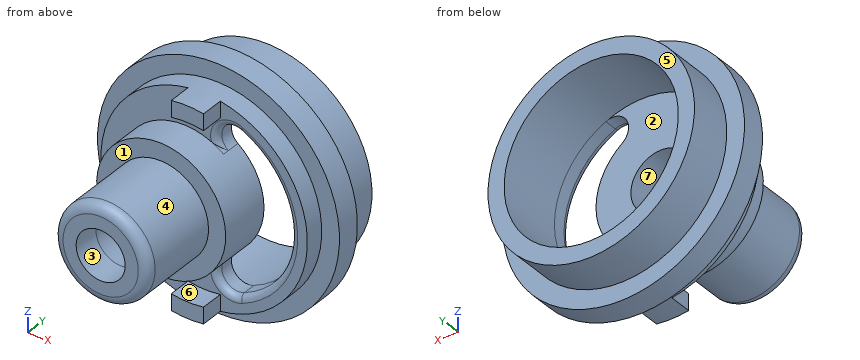
from build123d import *

# Parameters (mm, degrees)
SKETCH1_R              = 8.128
TOP_BODY_DEPTH         = 6.858
SKETCH2_R              = 5.08
ECCENTRIC_SLEEVE_DEPTH = 2.54
SKETCH3_R              = 3.724670389
ECCENTRIC_SHAFT_DEPTH  = 15.8242
SKETCH4_R              = 9.525
FLANGE_DEPTH           = 1.905
SKETCH5_R              = 6.858
TOP_HOLE_DEPTH         = 18.073240643
GROOVE_DEPTH           = 18.073240643
PINS_DEPTH             = 1.778
FILLET1_R              = 0.508
FILLET2_R              = 0.762


with BuildPart() as part:
    # Sketch1 → Top Body (new body)
    with BuildSketch(Plane(origin=(0, 0, 0), x_dir=(1, 0, 0), z_dir=(0, 1, 0))):
        with Locations(Location((0, 0, 0), (0, 0, 270))):
            Circle(SKETCH1_R)
    extrude(amount=TOP_BODY_DEPTH)

    # Sketch2 → Eccentric Sleeve (add)
    with BuildSketch(Plane.XZ):
        with Locations(Location((-1.4986, 0, 0), (0, 0, 90))):
            Circle(SKETCH2_R)
    extrude(amount=ECCENTRIC_SLEEVE_DEPTH)

    # Sketch3 → Eccentric Shaft (add)
    with BuildSketch(Plane(origin=(0, 6.858, 0), x_dir=(-1, 0, 0), z_dir=(0, 1, 0))):
        with Locations(Location((1.4986, 0, 0), (0, 0, 90))):
            Circle(SKETCH3_R)
    extrude(amount=-ECCENTRIC_SHAFT_DEPTH)

    # Sketch4 → Flange (add)
    with BuildSketch(Plane.XZ.offset(-1.524)):
        with Locations(Location((0, 0, 0), (0, 0, 270))):
            Circle(SKETCH4_R)
    extrude(amount=-FLANGE_DEPTH)

    # Sketch5 → Top Hole (cut, through all)
    with BuildSketch(Plane.XZ.offset(-1.524)):
        with Locations(Location((0, 0, 0), (0, 0, 270))):
            Circle(SKETCH5_R)
    extrude(amount=-TOP_HOLE_DEPTH, mode=Mode.SUBTRACT)

    # Sketch6 → Tapped Hole (revolve, cut)
    with BuildSketch(Plane.XY, mode=Mode.PRIVATE) as tapped_hole_sk:
        Polygon((0.8382, 1.524), (-1.4986, 1.524), (-1.4986, -8.9662), (0.4318, -8.9662), (0.4318, -6.859631692), (0.8382, -3.81), align=None)
    revolve(tapped_hole_sk.sketch.rotate(Axis((-1.4986, 5.365186462, 0), (0, -1, 0)), 180), axis=Axis((-1.4986, 5.365186462, 0), (0, -1, 0)), mode=Mode.SUBTRACT)

    # Sketch7 → Groove (cut, through all)
    with BuildSketch(Plane(origin=(0, 1.524, 0), x_dir=(-1, 0, 0), z_dir=(0, 1, 0))):
        with BuildLine():
            ThreePointArc((-2.805281279, 6.257999756), (-6.858, 0), (-2.805281279, -6.257999756))
            ThreePointArc((-2.805281279, -6.257999756), (-1.189982392, -5.741074463), (-1.528907797, -4.07928873))
            ThreePointArc((-1.528907797, -4.07928873), (-3.5814, 0), (-1.528907797, 4.07928873))
            ThreePointArc((-1.528907797, 4.07928873), (-1.189982392, 5.741074463), (-2.805281279, 6.257999756))
        make_face()
    extrude(amount=-GROOVE_DEPTH, mode=Mode.SUBTRACT)

    # Sketch8 → Pins (add)
    with BuildSketch(Plane.XZ):
        with BuildLine():
            Line((-1.27, 8.02816816), (-1.27, 6.739381574))
            ThreePointArc((-1.27, 6.739381574), (0, 6.858), (1.27, 6.739381574))
            Line((1.27, 6.739381574), (1.27, 8.02816816))
            ThreePointArc((1.27, 8.02816816), (0, 8.128), (-1.27, 8.02816816))
        make_face()
        with BuildLine():
            Line((1.27, -6.739381574), (1.27, -8.02816816))
            ThreePointArc((1.27, -8.02816816), (0, -8.128), (-1.27, -8.02816816))
            Line((-1.27, -8.02816816), (-1.27, -6.739381574))
            ThreePointArc((-1.27, -6.739381574), (0, -6.858), (1.27, -6.739381574))
        make_face()
    extrude(amount=PINS_DEPTH)

    # Fillet1
    # the kernel refuses this fillet: 0.508 mm, written as the material it takes off along each edge
    with BuildSketch(Plane(origin=(2.285784746, 0, -5.099110912), x_dir=(0.40905238828967766, 0, -0.9125109005565417), z_dir=(0.9125109005565417, 0, 0.40905238828967766))) as fillet1_piece_1_section:
        with BuildLine():
            CenterArc((1.27 + FILLET1_R, FILLET1_R), FILLET1_R, 180, 90)
            Line((1.27, FILLET1_R), (1.27, 0))
            Line((1.27, 0), (1.27 + FILLET1_R, 0))
        make_face()
    fillet1_piece_1 = revolve(axis=Axis((2.285784746, 0, -5.099110912), (0, 1, 0)), revolution_arc=224.939404777, mode=Mode.PRIVATE)
    fillet1_piece_1 = fillet1_piece_1 - Plane(origin=(-1.4986, 0.082765889, 0), x_dir=(0, 0, 1), z_dir=(0, 1, 0)) * Cylinder(5.08, 8, mode=Mode.PRIVATE)
    add(fillet1_piece_1, mode=Mode.SUBTRACT)
    with BuildSketch(Plane(origin=(0, 0, 0), x_dir=(0.40905238828967727, 0, 0.9125109005565418), z_dir=(-0.9125109005565418, 0, 0.40905238828967727))) as fillet1_piece_2:
        with BuildLine():
            CenterArc((6.858 + FILLET1_R, FILLET1_R), FILLET1_R, 180, 90)
            Line((6.858, FILLET1_R), (6.858, 0))
            Line((6.858, 0), (6.858 + FILLET1_R, 0))
        make_face()
    revolve(axis=Axis((0, 0, 0), (0, 1, 0)), revolution_arc=131.709357588, mode=Mode.SUBTRACT)
    with BuildSketch(Plane(origin=(2.285784746, 0, 5.099110912), x_dir=(0.355010429323337, 0, -0.9348623401718886), z_dir=(0.9348623401718886, 0, 0.355010429323337))) as fillet1_piece_3_section:
        with BuildLine():
            CenterArc((1.27 + FILLET1_R, FILLET1_R), FILLET1_R, 180, 90)
            Line((1.27, FILLET1_R), (1.27, 0))
            Line((1.27, 0), (1.27 + FILLET1_R, 0))
        make_face()
    fillet1_piece_3 = revolve(axis=Axis((2.285784746, 0, 5.099110912), (0, 1, 0)), revolution_arc=224.939404777, mode=Mode.PRIVATE)
    fillet1_piece_3 = fillet1_piece_3 - Plane(origin=(-1.4986, 0.254, 0), x_dir=(0, 0, 1), z_dir=(0, 1, 0)) * Cylinder(5.08, 8, mode=Mode.PRIVATE)
    add(fillet1_piece_3, mode=Mode.SUBTRACT)

    # Fillet2
    fillet2_edges = [part.edges().sort_by_distance(p)[0] for p in [
        (-1.4986, -8.9662, -3.724670389),
    ]]
    fillet(fillet2_edges, radius=FILLET2_R)


solid = part.part
Build history of the part. All positions in model axes, mm. Face numbers are marked on the shaded views. A direction names the side the tool comes from. Round coordinates to 2 decimals unless told otherwise and drop trailing zeros. Loops run counter-clockwise (first coordinate to the right, second up) from the corner with the lowest first, then second, coordinate; pieces in that order, holes last. Notation, with made-up numbers: (-30.5, 0) -> (11.5, 0) arc R27 cw to (11.5, 31) -> close; hole circle Ø9 at (-9, 80.25). An arc over 180 degrees is marked (long way). Answer in a Markdown table with one row per item.
Item 1: Saw through at B-B (z = 0). State how many separate pieces and enclosed holes the cut face has, and give its area (3 significant figures).
Answers below:
| item | result |
|---|---|
| separate pieces | 3 |
| enclosed holes | 0 |
| area | 65.9 mm² |
Item 2: Which spindle directions (+Z, -Z, +X, -X, +Y, -Y) get a long thin tool onto all of the face, cutting with end or side? Do the marked faces 1, 2 and 3. Say none if no direction does.
Answers below:
| item | result |
|---|---|
| face 1 | -Y |
| face 2 | +Y |
| face 3 | +Y, -Y |
Item 3: Pin check, flat tips, straight feed: pin 1 (0.6 mm diameter, centred on y = -0.5, z = -7.5, fed in from -X); pin 2 (11 mm diameter, centred on x = 0, z = 0, fed in from +Y); pin 3 (0.7 mm diameter, centred on x = -0.5, z = -7.5, fed in from -Y). Stop position of each tip, or through.
Answers below:
| item | result |
|---|---|
| pin 1 | stops at x = -1.27 |
| pin 2 | stops at y = 1.52 |
| pin 3 | stops at y = -1.78 |
Item 4: Mould opens along X. For the marked faces 4, 5, 6 and 7 say: +X half, -X half, draft (parallel to the pull), parting line (faces both ways), or undercut.
Answers below:
| item | result |
|---|---|
| face 4 | parting line |
| face 5 | draft |
| face 6 | undercut |
| face 7 | undercut |
Item 5: Saw through at D-D (z = 7.75). Write the cut outline in (x, y).
Answers below:
| item | result |
|---|---|
| outline | (-5.54, 1.52) -> (-2.45, 1.52) -> (-2.45, 0) -> (-1.27, 0) -> (-1.27, -1.78) -> (1.27, -1.78) -> (1.27, 0) -> (2.45, 0) -> (2.45, 1.52) -> (5.54, 1.52) -> (5.54, 3.43) -> (2.45, 3.43) -> (2.45, 6.86) -> (-2.45, 6.86) -> (-2.45, 3.43) -> (-5.54, 3.43) -> close |
Item 6: Saw through at A-A (y = -1.25). Write the cut outline in (x, z), and give its area (3 significant figures).
Answers below:
| item | result |
|---|---|
| outline | circle Ø10.16 at (-1.5, 0); (-1.27, -8.03) arc R8.13 ccw to (1.27, -8.03) -> (1.27, -6.74) arc R6.86 cw to (-1.27, -6.74) -> close; (-1.27, 6.74) arc R6.86 cw to (1.27, 6.74) -> (1.27, 8.03) arc R8.13 ccw to (-1.27, 8.03) -> close; hole circle Ø4.67 at (-1.5, 0) |
| area | 70.4 mm² |
Item 7: Drill centre lines: L1, parallel to Z at x = 1.5, y = 1; L2, parallel to X at y = 3.65, z = 0; L3, parallel to Z at x = 1.25, y = 3.5. Where is each one in solid material? Low to high. Write a range as [from, to].
Answers below:
| item | result |
|---|---|
| L1 | z = [-7.99, -6.1], [-4.1, 4.1], [6.1, 7.99] |
| L2 | x = [-8.13, -6.86], [6.86, 8.13] |
| L3 | z = [-8.03, -6.74], [6.74, 8.03] |
Item 8: Saw through at C-C (y = 5). Write the cut outline in (x, z).
Answers below:
| item | result |
|---|---|
| outline | circle Ø16.26 at (0, 0); hole circle Ø13.72 at (0, 0) |
